Here's how the part is built. I have some questions about the finished solid (model axes, mm). A direction names the side the tool comes from. Give positions to 0.01 mm unless a question says otherwise; leave off trailing zeros. Loops run counter-clockwise (first coordinate to the right, second up) from the corner with the lowest first, then second, coordinate; pieces in that order, holes last.
Q1. Will this pin go through, and if not, where does the flat tip stop? P1, Ø1, axis at y = 23, z = 8, coming from the +X side.
Q2. I need wall thicknesses on line 1 (Y direction, x = 1.25, z = -4); line 2 (Y direction, x = 8.25, z = -5.75); line 3 (Y direction, x = 4.5, z = 4). Which ranges of each line are inside material? Lowest first, please.
Q3. If we section it at C-C (x = 0): Please give me the cut outline in (y, z) (3 decimals), plus the area to 3 significant figures.
Q4. For faces 5 (the face through (0, 99.08, 0)), 6 (the face through (-1.424, 4.056, 4.521)), which set-ups out of +Z, -Z, +X, -X, +Y, -Y let a thin tool reach every point of the face, with its end or its side?
Q5. We'd pull the mould along Y, two halves only. Please class faces 1 (the face through (1, 9, 0)), 2 (the face through (6.21, 12.33, 3.23)), 3 (the face through (-7, 14.08, -2)), 4 (the face through (1, 8, 1)): +Y half, -Y half, draft (parallel to the pull), parting line (faces both ways), or undercut.
Q6. If we section it at D-D (y = 67.5): Please give me the cut outline in (x, z) (3 decimals), plus the area to 3 significant figures.
Q7. If we section it at A-A (z = -2.25): Please give me the cut outline in (x, y), plus the area to 3 significant figures.
Q8. If we section it at B-B (x = 3.75): Please give me the cut outline in (y, z).
from build123d import *

# Parameters (mm, degrees)
CUT_EXTRUDE1_DEPTH = 101.2883226


with BuildPart() as part:
    # Sketch1 → Revolve1 (revolve)
    with BuildSketch(Plane.XY, mode=Mode.PRIVATE) as revolve1_sk:
        Polygon((0, 0), (4.74, 0), (4.74, 8), (1, 8), (1, 10.53), (7, 10.53), (7, 14.08), (10.975, 14.08), (10.975, 99.08), (0, 99.08), align=None)
    revolve(revolve1_sk.sketch.rotate(Axis((0, 72.454564891, 0), (0, -1, 0)), 90), axis=Axis((0, 72.454564891, 0), (0, -1, 0)))

    # Sketch2 → Cut-Extrude1 (cut, through all)
    with BuildSketch(Plane(origin=(0, 99.08, 0), x_dir=(1, 0, 0), z_dir=(0, 1, 0))):
        with BuildLine():
            Line((-9.75, 5.038663017), (-9.75, -5.038663017))
            ThreePointArc((-9.75, -5.038663017), (-10.975, 0), (-9.75, 5.038663017))
        make_face()
        with BuildLine():
            Line((9.75, -5.038663017), (9.75, 5.038663017))
            ThreePointArc((9.75, 5.038663017), (10.975, 0), (9.75, -5.038663017))
        make_face()
    extrude(amount=-CUT_EXTRUDE1_DEPTH, mode=Mode.SUBTRACT)


solid = part.part
Check sheet entries:
1. P1: stops at x = 8.01
2. line 1: y = 0 to 8, 10.53 to 99.08
2. line 2: y = 14.08 to 99.08
2. line 3: y = 10.53 to 99.08
3. outline: (0, -4.74) - (8, -4.74) - (8, -1) - (10.53, -1) - (10.53, -7) - (14.08, -7) - (14.08, -10.975) - (99.08, -10.975) - (99.08, 10.975) - (14.08, 10.975) - (14.08, 7) - (10.53, 7) - (10.53, 1) - (8, 1) - (8, 4.74) - (0, 4.74) - close
3. area: 2,000 mm2
4. face 5: +Z, -Z, +X, -X, +Y
4. face 6: -Y
5. face 1: undercut
5. face 2: draft
5. face 3: -Y half
5. face 4: undercut
6. outline: (-9.75, -5.039) arc R10.975 ccw to (9.75, -5.039) - (9.75, 5.039) arc R10.975 ccw to (-9.75, 5.039) - close
6. area: 362 mm2
7. outline: (-9.75, 14.08) - (-6.63, 14.08) - (-6.63, 10.53) - (6.63, 10.53) - (6.63, 14.08) - (9.75, 14.08) - (9.75, 99.08) - (-9.75, 99.08) - close; (-4.17, 0) - (4.17, 0) - (4.17, 8) - (-4.17, 8) - close
7. area: 1,770 mm2
8. outline: (0, -2.9) - (8, -2.9) - (8, 2.9) - (0, 2.9) - close; (10.53, -5.91) - (14.08, -5.91) - (14.08, -10.31) - (99.08, -10.31) - (99.08, 10.31) - (14.08, 10.31) - (14.08, 5.91) - (10.53, 5.91) - close
